Verification items for the finished model (mm, model axes). Face numbers are marked on the shaded views. A direction names the side the tool comes from. Round coordinates to 2 decimals unless told otherwise and drop trailing zeros. Loops run counter-clockwise (first coordinate to the right, second up) from the corner with the lowest first, then second, coordinate; pieces in that order, holes last. Notation, with made-up numbers: (13.5, 12.25) -> (47.5, 12.25) arc R31 ccw to (47.5, 45.25) -> close; hole circle Ø1 at (87.5, -6). An arc over 180 degrees is marked (long way). Use a Markdown table: item, result. Add a question column.
```python
from build123d import *

# Parameters (mm, degrees)
F0_W     = 45
F0_H     = 35
F0_W_2   = 35
F0_H_2   = 45
F0_W_3   = 5
F0_H_3   = 5
F3_DEPTH = 2
F4_DEPTH = 20
F1_R     = 1.5
F5_DEPTH = 25
F2_R     = 1.5
F6_DEPTH = 25
F7_R     = 2


with BuildPart() as f3:
    # F0 (on Top) → F3 (new body)
    with BuildSketch(Plane.XY):
        with Locations((57.5, 17.5)):
            Rectangle(F0_W, F0_H)
        with Locations((17.5, 17.5)):
            Rectangle(F0_W_2, F0_H)
        with Locations((17.5, 57.5)):
            Rectangle(F0_W_2, F0_H_2)
        with Locations((-2.5, 17.5)):
            Rectangle(F0_W_3, F0_H)
        with Locations((17.5, -2.5)):
            Rectangle(F0_W_2, F0_H_3)
        Polygon((0, -5), (0, 0), (-5, 0), align=None)
    extrude(amount=-F3_DEPTH)

    # F0 (on Top) → F4 (join)
    with BuildSketch(Plane.XY):
        Polygon((0, -5), (0, 0), (-5, 0), align=None)
        with Locations((17.5, -2.5)):
            Rectangle(F0_W_2, F0_H_3)
        with Locations((-2.5, 17.5)):
            Rectangle(F0_W_3, F0_H)
    extrude(amount=F4_DEPTH)

    # F1 (on Front) → F5 (cut)
    with BuildSketch(Plane.XZ):
        with Locations((17.5, 10)):
            Circle(F1_R)
    extrude(amount=F5_DEPTH, mode=Mode.SUBTRACT)

    # F2 (on Right) → F6 (cut)
    with BuildSketch(Plane.YZ):
        with Locations((17.5, 10)):
            Circle(F2_R)
    extrude(amount=-F6_DEPTH, mode=Mode.SUBTRACT)

    # F7
    f7_edges = [f3.edges().sort_by_distance(p)[0] for p in [
        (16, -5, 10),
        (-5, 16, 10),
    ]]
    fillet(f7_edges, radius=F7_R)


solid = f3.part
```
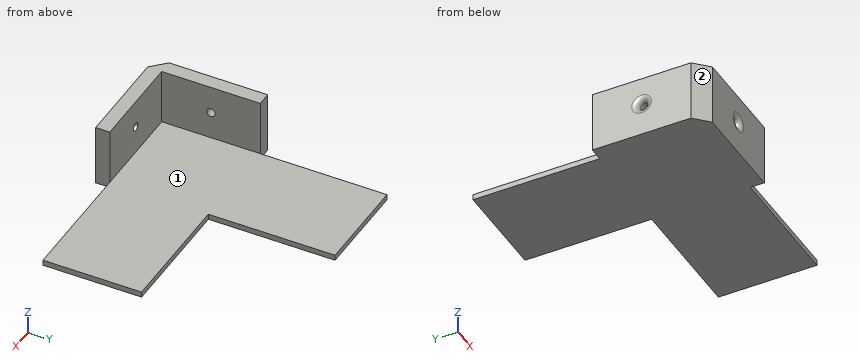
1) Thickness scan on line 1 (Z direction, x = -1.35, y = 17.5); line 2 (X direction, y = 7, z = 3). Record the ranges inside material, lowest first.
2) Go/stop test with flat-tipped pins: pin 1 (1 mm diameter, centred on y = 60, z = -1.5, fed in from +X); pin 2 (8 mm diameter, centred on y = 56.5, z = 6, fed in from -X); pin 3 (24 mm diameter, centred on x = 34, y = 52, fed in from +Z); pin 4 (1 mm diameter, centred on y = 66, z = -0.5, fed in from -X). Record where each tip stops, or that it passes through.
3) Sectioned sample at D-D on z = 2.25. Enter the section's corners in (x, y), then the cut area to 4 significant figures.
4) Sectioned sample at A-A on x = 17.5. Enter the section's corners in (y, z), then the cut area to 3 significant figures.
5) Sectioned sample at C-C on z = 10. Enter the section's corners in (x, y), then the cut area to 3 significant figures.
6) Access from +Z, -Z, +X, -X, +Y, -Y to the whole of each face (thin tool, end or side, straight path). Record for the marked faces 1 and 2.
Geometry results:
| question | item | result |
|---|---|---|
| 1 | line 1 | -2 to 8.5, 11.5 to 20 |
| 1 | line 2 | -5 to 0 |
| 2 | pin 1 | x = 35 |
| 2 | pin 2 | through |
| 2 | pin 3 | z = 0 |
| 2 | pin 4 | x = 0 |
| 3 | outline | (-5, 0) -> (0, -5) -> (35, -5) -> (35, 0) -> (0, 0) -> (0, 35) -> (-5, 35) -> close |
| 3 | area | 362.5 mm^2 |
| 4 | outline | (-5, -2) -> (80, -2) -> (80, 0) -> (0, 0) -> (0, 8.5) -> (-3, 8.5) arc R2 ccw to (-5, 6.5) -> close; (-5, 13.5) arc R2 ccw to (-3, 11.5) -> (0, 11.5) -> (0, 20) -> (-5, 20) -> close |
| 4 | area | 253 mm^2 |
| 5 | outline | (-5, 0) -> (0, -5) -> (14, -5) arc R2 ccw to (16, -3) -> (16, 0) -> (0, 0) -> (0, 16) -> (-3, 16) arc R2 ccw to (-5, 14) -> close; (-5, 21) arc R2 ccw to (-3, 19) -> (0, 19) -> (0, 35) -> (-5, 35) -> close; (19, -3) arc R2 ccw to (21, -5) -> (35, -5) -> (35, 0) -> (19, 0) -> close |
| 5 | area | 329 mm^2 |
| 6 | face 1 | +Z, +X, +Y |
| 6 | face 2 | +Z, -Z, -X, -Y |
